Can you work these out from the drawing? Everything is in mm from the part's minimum corner. A direction names the side the tool comes from. Coordinates: 2 decimals unless noted, no trailing zeros. Loops run counter-clockwise (first coordinate to the right, second up) from the corner with the lowest first, then second, coordinate; pieces in that order, holes last.
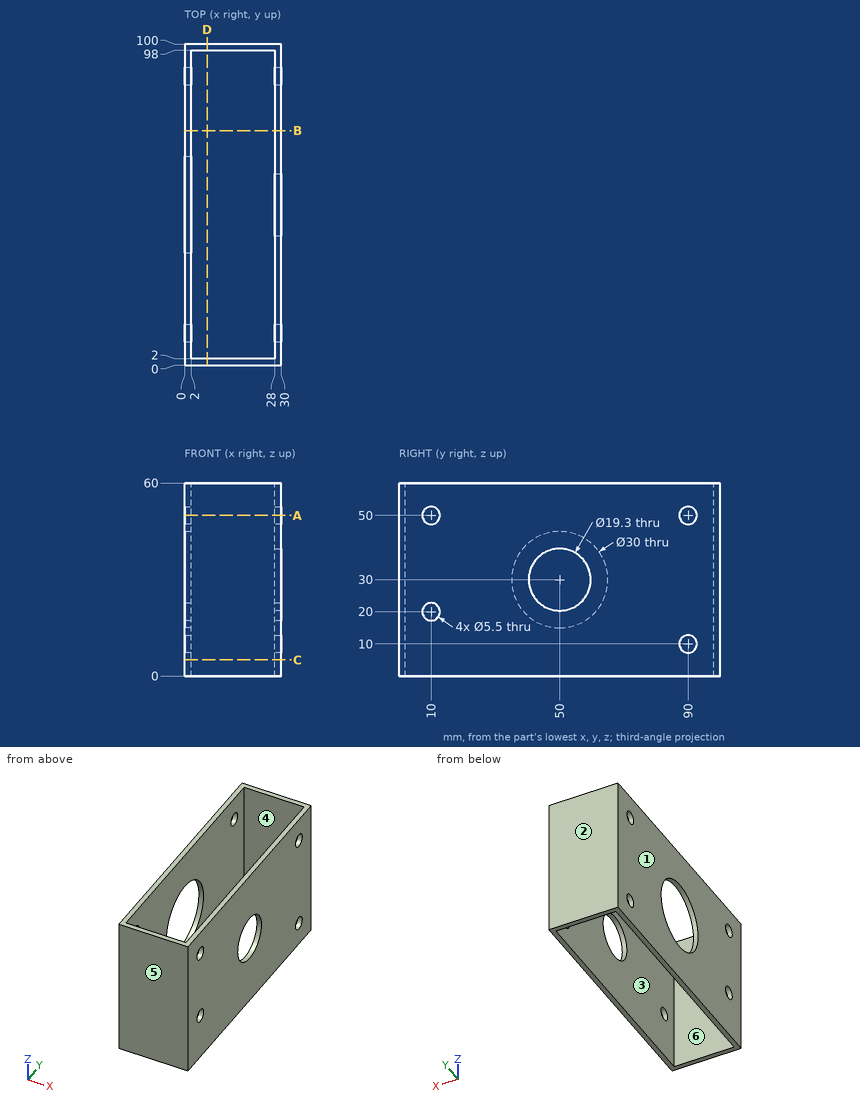
1) We'd pull the mould along X, two halves only. Please class the marked faces 1, 2, 3 and 4: released by +X, released by -X, zero draft, split by the parting line, or undercut.
2) Imagine slicing it at A-A on z = 50. List the corners of the cut face in (x, y) for me, plus the area to 3 significant figures.
3) Imagine slicing it at B-B on y = 73. List the corners of the cut face in (x, z) for me.
4) Imagine slicing it at D-D on x = 7. List the corners of the cut face in (y, z) for me.
5) If I drill on L1, parallel to X at y = 90, z = 57; L2, parallel to Y at x = 0.7, z = 10; L3, parallel to Y at x = 23, z = 56.5, over which ranges is the centre line in solid material (lowest first)?
6) For the marked faces 5 and 6, which set-ups out of +Z, -Z, +X, -X, +Y, -Y let a thin tool reach every point of the face, with its end or its side?
7) Imagine slicing it at C-C on z = 5. List the corners of the cut face in (x, y) for me, plus the area to 3 significant figures.
8) Will this pin go through, and if not, where does the flat tip stop? pin 1 (1.5 mm diameter, centred on y = 36, z = 46.5, fed in from -X).
Solved:
1. face 1: released by -X
1. face 2: zero draft
1. face 3: undercut
1. face 4: undercut
2. outline: (0, 0) - (30, 0) - (30, 7.25) - (28, 7.25) - (28, 2) - (2, 2) - (2, 7.25) - (0, 7.25) - close; (0, 12.75) - (2, 12.75) - (2, 87.25) - (0, 87.25) - close; (0, 92.75) - (2, 92.75) - (2, 98) - (28, 98) - (28, 92.75) - (30, 92.75) - (30, 100) - (0, 100) - close; (28, 12.75) - (30, 12.75) - (30, 87.25) - (28, 87.25) - close
2. area: 460 mm2
3. outline: (0, 0) - (2, 0) - (2, 60) - (0, 60) - close; (28, 0) - (30, 0) - (30, 60) - (28, 60) - close
4. outline: (0, 0) - (2, 0) - (2, 60) - (0, 60) - close; (98, 0) - (100, 0) - (100, 60) - (98, 60) - close
5. L1: x = 0 to 2, 28 to 30
5. L2: y = 0 to 87.25, 92.75 to 100
5. L3: y = 0 to 2, 98 to 100
6. face 5: +Z, -Z, +X, -X, -Y
6. face 6: +Z, -Z
7. outline: (0, 0) - (30, 0) - (30, 100) - (0, 100) - close; hole (2, 2) - (28, 2) - (28, 98) - (2, 98) - close
7. area: 504 mm2
8. pin 1: stops at x = 0
